Verification items for the finished model (mm, model axes). A direction names the side the tool comes from. Coordinates: 2 decimals unless noted, no trailing zeros. Write each loop counter-clockwise with the first axis right and the second up, starting at its lowest first coordinate (ties: lowest second). Pieces come first, ordered by that corner, then holes. Notation, with made-up numbers: M 38.5,16.5 L 79.5,16.5 A35 ccw 79.5,54.5 Z; hole C 61,-39.5 d6. An arc over 180 degrees is marked long. Answer in a Markdown table with one row per item.
from build123d import *

# Parameters (mm, degrees)
IZIM1_W                     = 44
IZIM1_H                     = 25
Y_KSEKLIK_EKSTR_ZYON1_DEPTH = 2
IZIM3_W                     = 42
IZIM3_H                     = 25
Y_KSEKLIK_EKSTR_ZYON2_DEPTH = 2
IZIM5_W                     = 38
IZIM5_H                     = 21
KES_EKSTR_ZYON1_DEPTH       = 2


with BuildPart() as part:
    # Çizim1 → Yükseklik-Ekstrüzyon1 (new body)
    with BuildSketch(Plane.XY):
        Rectangle(IZIM1_W, IZIM1_H)
    extrude(amount=Y_KSEKLIK_EKSTR_ZYON1_DEPTH)

    # Çizim3 → Yükseklik-Ekstrüzyon2 (add)
    with BuildSketch(Plane.XY.offset(2)):
        Rectangle(IZIM3_W, IZIM3_H)
    extrude(amount=Y_KSEKLIK_EKSTR_ZYON2_DEPTH)

    # Çizim5 → Kes-Ekstrüzyon1 (cut)
    with BuildSketch(Plane.XY.offset(4)):
        Rectangle(IZIM5_W, IZIM5_H)
    extrude(amount=-KES_EKSTR_ZYON1_DEPTH, mode=Mode.SUBTRACT)


solid = part.part
1) Tool access check on faces 1 (the face through (21.5, 0.2, 2)), 2 (the face through (0, -10.5, 3)), 3 (the face through (-22, 0, 1)), 4 (the face through (-21.5, 0.2, 2)). Record the directions out of +Z, -Z, +X, -X, +Y, -Y that give a thin tool (end or side, any length) a straight path to the whole face; none if there is none.
Response values:
| item | result |
|---|---|
| face 1 | +Z, +X, +Y, -Y |
| face 2 | +Z |
| face 3 | +Z, -Z, -X, +Y, -Y |
| face 4 | +Z, -X, +Y, -Y |
2) Release check for a two-part mould opening along Y. For faces 5 (the face through (22, 0, 1)), 6 (the face through (0, -12.5, 2)), 7 (the face through (-19, 0, 3)) record: +Y half, -Y half, draft (parallel to the pull), parting line (faces both ways), or undercut.
Response values:
| item | result |
|---|---|
| face 5 | draft |
| face 6 | -Y half |
| face 7 | undercut |
3) Thickness scan on L1, parallel to X at y = -4, z = 2.1; L2, parallel to Y at x = -7, z = 2.6; L3, parallel to Z at x = 5, y = 2.75. Record the ranges inside material, lowest first. Write a range as [from, to].
Response values:
| item | result |
|---|---|
| L1 | x = [-21, -19], [19, 21] |
| L2 | y = [-12.5, -10.5], [10.5, 12.5] |
| L3 | z = [0, 2] |
4) Sectioned sample at C-C (x = -3). Record the cut outline in (y, z), then the cut area to 3 significant figures.
Response values:
| item | result |
|---|---|
| outline | M -12.5,0 L 12.5,0 L 12.5,4 L 10.5,4 L 10.5,2 L -10.5,2 L -10.5,4 L -12.5,4 Z |
| area | 58.0 mm² |
5) Sectioned sample at B-B (z = 3.4). Record the cut outline in (x, y).
Response values:
| item | result |
|---|---|
| outline | M -21,-12.5 L 21,-12.5 L 21,12.5 L -21,12.5 Z; hole M -19,-10.5 L 19,-10.5 L 19,10.5 L -19,10.5 Z |
6) Sectioned sample at A-A (y = -3.75). Record the cut outline in (x, z).
Response values:
| item | result |
|---|---|
| outline | M -22,0 L 22,0 L 22,2 L 21,2 L 21,4 L 19,4 L 19,2 L -19,2 L -19,4 L -21,4 L -21,2 L -22,2 Z |
7) Depth check by flat-ended pin: pin 1 (1 mm diameter, centred on y = -2, z = 3.5, fed in from -X); pin 2 (0.5 mm diameter, centred on x = -21.5, y = 0, fed in from +Z). Enter the tip coordinate at first touch or a pass-through.
Response values:
| item | result |
|---|---|
| pin 1 | stops at x = -21 |
| pin 2 | stops at z = 2 |
